Answer from the drawing. Dimensions are ordinates in mm from the lowest x, y and z of the part. A direction names the side the tool comes from. Round coordinates to 2 decimals unless told otherwise and drop trailing zeros. Write each loop counter-clockwise with the first axis right and the second up, starting at its lowest first coordinate (ties: lowest second). Pieces come first, ordered by that corner, then holes. Notation, with made-up numbers: M -29.5,59.5 L -23.5,59.5 A29 cw -23.5,96.5 Z; hole C 50,80.25 d8. An arc over 180 degrees is marked long. Answer as CSV lines item,"result". Start each with the question number.
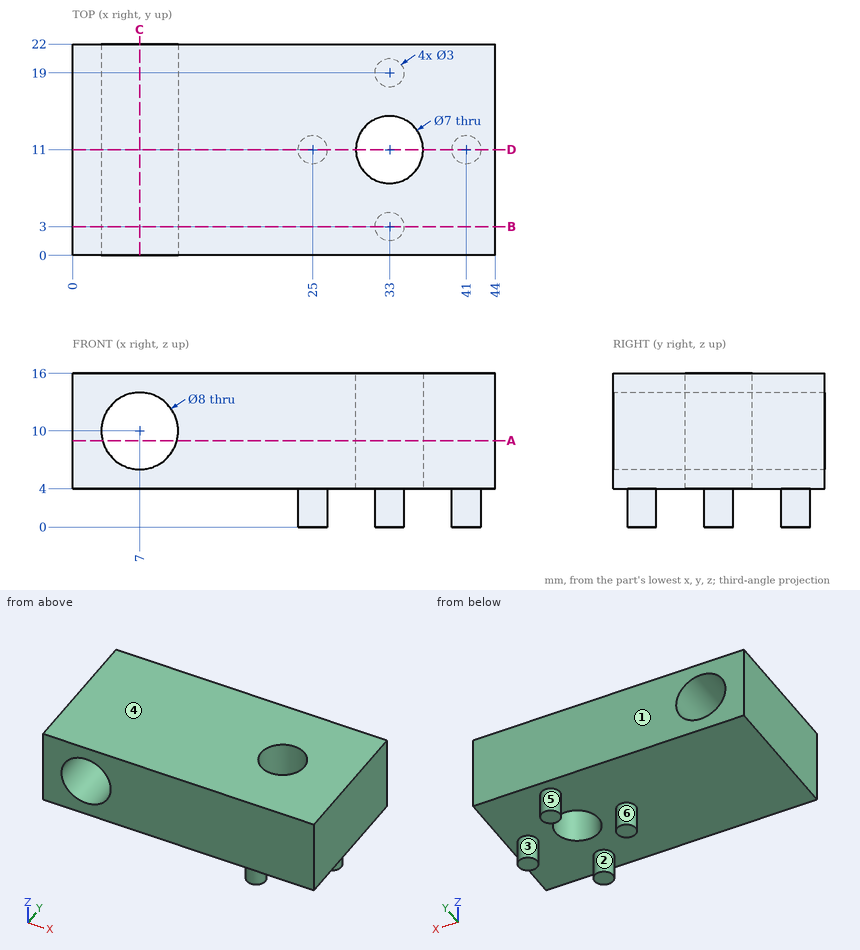
Q1. Find section A-A (z = 9). Determine the outline of the cut face in (x, y), plus the area to 3 significant figures.
Q2. Straight lines are drawn through the part: L1, parallel to Y at x = 33, z = 10.75; L2, parallel to X at y = 16, z = 10; L3, parallel to X at y = 12.5, z = 8.5. For each, find the intervals that lie inside material, in ascending order.
Q3. Each of these flat-tipped pins is pushed along its axis until it touches: P1, Ø2, axis at x = 5, z = 3.5, coming from the +Y side; P2, Ø4, axis at x = 7.5, y = 13.5, coming from the -Z side. Where does it stop, or does it pass through?
Q4. The mould has two halves that part along X. Classify the marked faces 3, 4, 5 and 6: +X half, -X half, draft (parallel to the pull), parting line (faces both ways), or undercut.
Q5. Find section C-C (x = 7). Determine the outline of the cut face in (y, z).
Q6. Find section D-D (y = 11). Determine the outline of the cut face in (x, z).
Q7. Find section B-B (y = 3). Determine the outline of the cut face in (x, z).
Q8. For the marked faces 1 and 2, determine the directions among +Z, -Z, +X, -X, +Y, -Y from which every point of the face is accessible in a straight line to the end or side of a thin tool.
Reported:
1,outline,"M 0,0 L 3.13,0 L 3.13,22 L 0,22 Z; M 10.87,0 L 44,0 L 44,22 L 10.87,22 Z; hole C 33,11 d7"
1,area,"759 mm2"
2,L1,"y = 0 to 7.5, 14.5 to 22"
2,L2,"x = 0 to 3, 11 to 44"
2,L3,"x = 0 to 3.29, 10.71 to 29.84, 36.16 to 44"
3,P1,"stops at y = 22"
3,P2,"stops at z = 4"
4,face 3,"undercut"
4,face 4,"draft"
4,face 5,"parting line"
4,face 6,"undercut"
5,outline,"M 0,4 L 22,4 L 22,6 L 0,6 Z; M 0,14 L 22,14 L 22,16 L 0,16 Z"
6,outline,"M 0,4 L 23.5,4 L 23.5,0 L 26.5,0 L 26.5,4 L 29.5,4 L 29.5,16 L 0,16 Z; M 36.5,4 L 39.5,4 L 39.5,0 L 42.5,0 L 42.5,4 L 44,4 L 44,16 L 36.5,16 Z; hole C 7,10 d8"
7,outline,"M 0,4 L 31.5,4 L 31.5,0 L 34.5,0 L 34.5,4 L 44,4 L 44,16 L 0,16 Z; hole C 7,10 d8"
8,face 1,"+Z, -Z, +X, -X, +Y"
8,face 2,"-Z"
